Autodesk Inventor part; units mm, degrees
ref_plane "YZ Plane" through (0, 0, 0) normal (1, 0, 0) x (0, 1, 0)
ref_plane "XZ Plane" through (0, 0, 0) normal (0, 1, 0) x (-1, 0, 0)
ref_plane "XY Plane" through (0, 0, 0) normal (0, 0, 1) x (1, 0, 0)
sketch "Sketch4" plane through (0, 0, 0) normal (0, 0, 1) x (1, 0, 0)
  line L0 (-10.5, 0) -> (10.5, 0)
  line L1 (0, -3.3) -> (0, 19.8)
  line L2 (-7.5, 0) -> (7.5, 0)
  line L3 (7.5, 0) -> (7.5, 16.5)
  line L4 (7.5, 16.5) -> (-7.5, 16.5)
  line L5 (-7.5, 16.5) -> (-7.5, 0)
  circle A0 centre (0, 10) radius 2.5
  point P0 (0, 0)
  dimension "d0" = 7.5
  dimension "d1" = 7.5
  dimension "d2" = 16.5
  dimension "d3" = 5
  dimension "d4" = 6.5
extrude "Extrusion1" add sketch "Sketch4" against normal blind 15.9 contours L5 L4 L1 A0 L0 | L1 A0 L4 L3 L0
fillet "Fillet1" radius 7.5 2 edges at (7.5, 16.5, -7.95) (-7.5, 16.5, -7.95)
sketch "Sketch13" plane through (7.5, 9, 0) normal (1, 0, 0) x (0, 0, -1)
  line L0 (0, -12.3) -> (0, 10.8)
  line L1 (19.08, -9) -> (-3.18, -9)
  line L2 (0, -9) -> (0, 0)
  line L3 (0, 7.5) -> (15.9, 7.5)
  line L4 (0, -9) -> (2.7, -9)
  line L5 (2.7, -9) -> (2.7, 7.5)
  line L6 (2.7, 7.5) -> (0, 7.5)
  line L7 (0, 7.5) -> (0, -9)
  line L8 (15.9, -9) -> (15.9, 0)
  line L9 (15.9, -9) -> (13.2, -9)
  line L10 (13.2, -9) -> (13.2, 7.5)
  line L11 (13.2, 7.5) -> (15.9, 7.5)
  line L12 (15.9, 7.5) -> (15.9, -9)
  line L13 (6.6, -9) -> (9.3, -9)
  line L14 (9.3, -9) -> (9.3, 7.5)
  line L15 (9.3, 7.5) -> (6.6, 7.5)
  line L16 (6.6, 7.5) -> (6.6, -9)
  dimension "d47" = 2.7
  dimension "d48" = 2.7
  dimension "d49" = 2.7
  dimension "d50" = 15.9
  dimension "d51" = 3.9
  dimension "d52" = 3.9
extrude "Extrusion8" cut sketch "Sketch13" against normal through all contours L5 L3 L16 L1 | L14 L3 L10 L1
sketch "Sketch14" plane through (-7.5, 0, -6.6) normal (0, -1, 0) x (1, 0, 0)
  line L0 (0, 6.6) -> (15, 6.6)
  line L1 (15, -9.3) -> (0, -9.3)
  line L2 (15, 6.6) -> (0, 6.6)
  line L3 (0, 6.6) -> (0, -9.3)
  line L4 (0, -9.3) -> (15, -9.3)
  line L5 (15, -9.3) -> (15, 6.6)
  point P0 (7.5, 6.6)
extrude "Extrusion9" add sketch "Sketch14" along normal blind 4
sketch "Sketch15" plane through (0, 0, 0) normal (0, 0, 1) x (1, 0, 0)
  point P0 (0, 0)
sketch "Sketch16" plane through (0, 0, 0) normal (0, 0, 1) x (1, 0, 0)
  line L0 (-7.5, 9) -> (-7.5, -4)
  line L1 (-7.5, -4) -> (7.5, -4)
  line L2 (7.5, -4) -> (7.5, -24)
  line L3 (7.5, -24) -> (-7.5, -24)
  line L4 (-7.5, -24) -> (-7.5, -4)
  line L5 (7.5, -15) -> (5.5, -24)
  line L6 (-7.5, -15) -> (-5.5, -24)
  point P0 (0, 0)
  dimension "d57" = 15
  dimension "d58" = 20
  dimension "d59" = 9
  dimension "d60" = 2
  dimension "d61" = 2
  dimension "d62" = 9
extrude "Extrusion10" add sketch "Sketch16" against normal blind 15.9 contours L1 L2 L5 L3 L6 L4
properties part number "mountBrio"
The model under review builds one solid part; all positions refer to its coordinate system, in mm. A direction names the side the tool comes from. Round coordinates to 2 decimals unless told otherwise and drop trailing zeros. Loops run counter-clockwise (first coordinate to the right, second up) from the corner with the lowest first, then second, coordinate; pieces in that order, holes last. Notation, with made-up numbers: (36, 77.5) - (90, 77.5) arc R26 ccw to (90, 103.5) - close; hole circle Ø1 at (84, 41). An arc over 180 degrees is marked (long way). Use a Markdown table: item, result. Add a question column.
Q1. Add section A-A (y = 3.5). State the section outline as (x, z) points, plus the area to 4 significant figures.
Q2. Machinability: for faces 1 (the face through (5.245, 14.361, -14.569)), 2 (the face through (0, 7, -6.6)), which of the approach directions +Z, -Z, +X, -X, +Y, -Y give a long, thin tool a straight path to every point of the face, cutting with its end or side? Answer none if there is none.
Q3. For probe 1 along Z at (x, y) = (-2.5, 4); probe 2 along Y at (x, z) = (0, -7.55); probe 3 along Y at (x, z) = (4, -11), list the stretches that pass through material, from the lowest coordinate up.
Q4. Add section C-C (x = 0.5). State the section outline as (y, z) points.
Q5. Insertion check: pin 1 Ø3 at (x, y) = (0, 10) entering from -Z; pin 2 Ø1.9 at (x, z) = (-1.5, -11.5) entering from +Y; pin 3 Ø3 at (x, z) = (3, -6) entering from +Y. Each pin has a flat end and moves straight along its axis. Give the tip position at first contact, or say it passes through.
Q6. The part is to be moulded in two halves that separate along X. For faces 3 (the face through (0, -3, 0)), 4 (the face through (-0.54, 7.56, -7.93)), 5 (the face through (-6.514, -19.437, -7.839)), 6 (the face through (-0.54, 7.56, -14.53)), say which applies: pulls with the +X half, pulls with the -X half, needs draft (parallel to the pull), parting line crosses it, or undercut.
Q7. Add section D-D (y = 10). State the section outline as (x, z) points.
Worked answers:
| question | item | result |
|---|---|---|
| 1 | outline | (-7.5, -15.9) - (7.5, -15.9) - (7.5, -13.2) - (-7.5, -13.2) - close; (-7.5, -9.3) - (7.5, -9.3) - (7.5, -6.6) - (-7.5, -6.6) - close; (-7.5, -2.7) - (7.5, -2.7) - (7.5, 0) - (-7.5, 0) - close |
| 1 | area | 121.5 mm² |
| 2 | face 1 | +Z, -Z, +X, +Y |
| 2 | face 2 | +X, -X, +Y |
| 3 | probe 1 | -15.9 to -13.2, -9.3 to -6.6, -2.7 to 0 |
| 3 | probe 2 | -24 to 7.5, 12.5 to 16.5 |
| 3 | probe 3 | -24 to 0 |
| 4 | outline | (-24, -15.9) - (7.55, -15.9) - (7.55, -13.2) - (0, -13.2) - (0, -9.3) - (7.55, -9.3) - (7.55, -6.6) - (0, -6.6) - (0, -2.7) - (7.55, -2.7) - (7.55, 0) - (-24, 0) - close; (12.45, -15.9) - (16.48, -15.9) - (16.48, -13.2) - (12.45, -13.2) - close; (12.45, -9.3) - (16.48, -9.3) - (16.48, -6.6) - (12.45, -6.6) - close; (12.45, -2.7) - (16.48, -2.7) - (16.48, 0) - (12.45, 0) - close |
| 5 | pin 1 | through |
| 5 | pin 2 | y = 0 |
| 5 | pin 3 | y = 16.32 |
| 6 | face 3 | needs draft |
| 6 | face 4 | undercut |
| 6 | face 5 | pulls with the -X half |
| 6 | face 6 | undercut |
| 7 | outline | (-7.43, -15.9) - (-2.5, -15.9) - (-2.5, -13.2) - (-7.43, -13.2) - close; (-7.43, -9.3) - (-2.5, -9.3) - (-2.5, -6.6) - (-7.43, -6.6) - close; (-7.43, -2.7) - (-2.5, -2.7) - (-2.5, 0) - (-7.43, 0) - close; (2.5, -15.9) - (7.43, -15.9) - (7.43, -13.2) - (2.5, -13.2) - close; (2.5, -9.3) - (7.43, -9.3) - (7.43, -6.6) - (2.5, -6.6) - close; (2.5, -2.7) - (7.43, -2.7) - (7.43, 0) - (2.5, 0) - close |
